Model file for the job. Use its own axes, mm. A direction names the side the tool comes from. Give positions to 0.01 mm unless a question says otherwise; leave off trailing zeros. Order: outer loops, then holes, each group sorted by start corner. A loop starts at its lowest first (then second) coordinate and runs counter-clockwise, first axis right, second up. Notation, with made-up numbers: (41.5, 49) - (74.5, 49) arc R26 cw to (74.5, 65) - close; hole circle Ø4 at (-32.5, 81). An arc over 180 degrees is marked (long way). Return JSON: item names as keys, results as strings. Group by question number.
Autodesk Inventor part; units mm, degrees
ref_plane "YZ Plane" through (0, 0, 0) normal (1, 0, 0) x (0, 1, 0)
ref_plane "XZ Plane" through (0, 0, 0) normal (0, 1, 0) x (-1, 0, 0)
ref_plane "XY Plane" through (0, 0, 0) normal (0, 0, 1) x (1, 0, 0)
sketch "Sketch1" plane through (0, 0, 0) normal (0, 0, 1) x (1, 0, 0)
  line L0 (0, 0) -> (311.15, 0)
  line L1 (311.15, 0) -> (311.15, 152.4)
  line L2 (311.15, 152.4) -> (0, 152.4)
  line L3 (0, 152.4) -> (0, 0)
  dimension "d0" = 311.15
  dimension "d1" = 152.4
extrude "Plate1" add sketch "Sketch1" along normal blind 1.5875
sketch "Sketch2" plane through (309.5625, 0, 1.5875) normal (1, 0, 0) x (0, 1, 0)
  line L0 (152.4, 0) -> (0, 0)
  line L1 (0, 0) -> (0, -101.6)
  line L2 (0, -101.6) -> (152.4, -101.6)
  line L3 (152.4, -101.6) -> (152.4, 0)
edge flange "Flange1" height 101.6 angle 90 thickness 1.5875 bend radius 1.5875 thickness toward (1, 0, 0) relief straight relief width 1.5875 relief depth 0.7937 corner gap 1.5875 corner form 0 edges at (311.15, 76.2, 0) (0, 76.2, 0) wall of the first edge with corners at (309.5625, 152.4, 1.5875) (309.5625, 0, 1.5875) (309.5625, 0, -100.0125) (309.5625, 152.4, -100.0125)
bend "Bend1"
corner "Corner1"
sketch "Sketch3" plane through (311.15, 0, -100.0125) normal (1, 0, 0) x (0, 0, -1)
  circle A0 centre (-73.025, 19.05) radius 2.54
  circle A1 centre (-25.4, 19.05) radius 2.54
  line L0 (0, 152.4) -> (0, 0)
  line L1 (-98.425, 152.4) -> (-98.425, 0)
  line L2 (0, 0) -> (-98.425, 0)
  point P0 (-100.0125, 0)
  dimension "d13" = 5.08
  dimension "d14" = 5.08
  dimension "d15" = 25.4
  dimension "d16" = 25.4
  dimension "d17" = 19.05
  dimension "d18" = 19.05
extrude "Extrusion1" cut sketch "Sketch3" against normal up to surface (311.15 mm away)
equation "\"d3\" = BendReliefWidth"
equation "\"d4\" = BendReliefDepth"
equation "\"d5\" = MinimumRemnant"
equation "\"d6\" = BendRadius"
equation "\"d9\" = BendRadius"
equation "\"d10\" = CornerReliefSize"
equation "\"d11\" = GapSize"
equation "\"d12\" = JacobiRadiusSize"
equation "\"BendRadius\" = Thickness"
equation "\"BendReliefWidth\" = Thickness"
equation "\"BendReliefDepth\" = 0.5 * Thickness"
equation "\"CornerReliefSize\" = 4 * Thickness"
equation "\"MinimumRemnant\" = 2 * Thickness"
equation "\"TransitionRadius\" = BendRadius"
equation "\"JacobiRadiusSize\" = Thickness"
equation "\"GapSize\" = Thickness"
equation "\"d2\" = BendRadius"
properties part number "Chute"
(1) Pull direction X, two halves, no side cores. Call faces 3 (the face through (153, 77, 1.588)), 4 (the face through (0, 77, -51)), 5 (the face through (1.588, 77, -50)): released by +X, released by -X, zero draft, split by the parting line, or undercut.
(2) 3-axis set-ups, long thin cutter, end or side, ignore diameter. For faces 1 (the face through (311.15, 75, -51)), 2 (the face through (153, 77, 0)): which of +Z, -Z, +X, -X, +Y, -Y reach the whole face in a straight line?
(3) Slice it at A-A (z = -38.5). Give the cut face in (x, y).
(4) Slice it at C-C (x = 236). Give the cut face in (y, z), and give its area (3 significant figures).
(5) Drill centre lines: L1, parallel to X at y = 57, z = -24.5; L2, parallel to Z at x = 1, y = 19; L3, parallel to Z at x = 189, y = 24.5. Where is each one in solid material? Low to high.
Result set:
{
 "1": {"face 3": "zero draft", "face 4": "released by -X", "face 5": "undercut"},
 "2": {"face 1": "+Z, -Z, +X, +Y, -Y", "face 2": "-Z, +Y, -Y"},
 "3": {"outline": "(0, 0) - (1.59, 0) - (1.59, 152.4) - (0, 152.4) - close; (309.56, 0) - (311.15, 0) - (311.15, 152.4) - (309.56, 152.4) - close"},
 "4": {"outline": "(0, 0) - (152.4, 0) - (152.4, 1.59) - (0, 1.59) - close", "area": "242 mm²"},
 "5": {"L1": "x = 0 to 1.59, 309.56 to 311.15", "L2": "z = -100.01 to -77.15, -72.07 to -29.53, -24.45 to 0.73", "L3": "z = 0 to 1.59"}
}
